from build123d import *

# Parameters (mm, degrees)
HUB_ENDPLATE_AXIAL_CLEARANCE_SHIM_H0P65_START = 3
SKETCH1_R                                     = 14
SKETCH1_R_2                                   = 7.025
HUB_ENDPLATE_AXIAL_CLEARANCE_SHIM_H0P65_DEPTH = 0.65
SKETCH2_R                                     = 1.4
FOUR_D2P8_PCD22_DEPTH                         = 20.809656736


with BuildPart() as part:
    # Sketch1 → Hub_Endplate_Axial_Clearance_Shim_H0p65 (new body)
    with BuildSketch(Plane.XY.offset(HUB_ENDPLATE_AXIAL_CLEARANCE_SHIM_H0P65_START)):
        Circle(SKETCH1_R)
        Circle(SKETCH1_R_2, mode=Mode.SUBTRACT)
    extrude(amount=HUB_ENDPLATE_AXIAL_CLEARANCE_SHIM_H0P65_DEPTH)

    # Sketch2 → Four_D2p8_PCD22 (cut, through all)
    with BuildSketch(Plane.XY.offset(3.65)):
        with Locations((7.778174593, 7.778174593)):
            Circle(SKETCH2_R)
        with Locations((-7.778174593, 7.778174593)):
            Circle(SKETCH2_R)
        with Locations((-7.778174593, -7.778174593)):
            Circle(SKETCH2_R)
        with Locations((7.778174593, -7.778174593)):
            Circle(SKETCH2_R)
    extrude(amount=-FOUR_D2P8_PCD22_DEPTH, mode=Mode.SUBTRACT)


solid = part.part
The listing builds one solid part. Answer for the finished solid, in the listing's coordinates (mm). Round coordinates to 2 decimals unless told otherwise and drop trailing zeros. Order: outer loops, then holes, each group sorted by start corner. A loop starts at its lowest first (then second) coordinate and runs counter-clockwise, first axis right, second up. Notation, with made-up numbers: M 46.5,-27.5 L 82.5,-27.5 A16 cw 82.5,-12.5 Z; hole C 41.25,14.25 d8. An arc over 180 degrees is marked long. Answer in a Markdown table with one row per item. Add a question column.
1) The part is cut by section A-A on x = 0. Determine the outline of the cut face in (y, z) (3 decimals).
2) Consider line 1 along Y through (x, z) = (0, 3.2) (3 decimals); line 2 along Y through (x, z) = (8.75, 3.3); line 3 along Y through (x, z) = (-9, 3.45). Determine where each line is inside the solid, lowest interval first. Write a range as from..to.
3) Determine the mould class of faces 1 (the face through (-6.4, 3.3, 3)), 2 (the face through (12.932, -5.362, 3.32)), 3 (the face through (8.424, 6.536, 3.33)), 4 (the face through (9.071, -8.314, 3.33)) for opening direction Y: pulls with the +Y half, pulls with the -Y half, needs draft (parallel to the pull), parting line crosses it, or undercut.
4) The part is cut by section D-D on x = -10.75. Determine the outline of the cut face in (y, z).
5) Flat-ended cylindrical pins translate along their axes: pin 1 Ø3 at (x, y) = (7.78, -7.78) entering from +Z; pin 2 Ø2 at (x, y) = (7.78, 7.78) entering from +Z. Find the tip coordinate at first contact, or state that the pin passes through.
6) The part is cut by section C-C on z = 3.35. Determine the outline of the cut face in (x, y) (3 decimals).
Findings below:
| question | item | result |
|---|---|---|
| 1 | outline | M -14,3 L -7.025,3 L -7.025,3.65 L -14,3.65 Z; M 7.025,3 L 14,3 L 14,3.65 L 7.025,3.65 Z |
| 2 | line 1 | y = -14..-7.025, 7.025..14 |
| 2 | line 2 | y = -10.93..-8.79, -6.77..6.77, 8.79..10.93 |
| 2 | line 3 | y = -10.72..-8.46, -7.09..7.09, 8.46..10.72 |
| 3 | face 1 | needs draft |
| 3 | face 2 | parting line crosses it |
| 3 | face 3 | undercut |
| 3 | face 4 | undercut |
| 4 | outline | M -8.97,3 L 8.97,3 L 8.97,3.65 L -8.97,3.65 Z |
| 5 | pin 1 | stops at z = 3.65 |
| 5 | pin 2 | passes through |
| 6 | outline | C 0,0 d28; hole C -7.778,-7.778 d2.8; hole C -7.778,7.778 d2.8; hole C 0,0 d14.05; hole C 7.778,-7.778 d2.8; hole C 7.778,7.778 d2.8 |
